```python
from build123d import *

# Parameters (mm, degrees)
SKETCH1_R           = 5.75
BOSS_EXTRUDE1_DEPTH = 7
CUT_EXTRUDE1_DEPTH  = 7
FILLET1_R           = 1
FILLET2_R           = 1
FILLET3_R           = 1
FILLET4_R           = 1
CUT_EXTRUDE2_DEPTH  = 0.5


with BuildPart() as part:
    # Sketch1 → Boss-Extrude1 (new body)
    with BuildSketch(Plane(origin=(0, 0, 0), x_dir=(1, 0, 0), z_dir=(0, 1, 0))):
        with BuildLine():
            Line((-27.5, -15), (27.5, -15))
            ThreePointArc((27.5, -15), (34.571067812, -12.071067812), (37.5, -5))
            Line((37.5, -5), (37.5, 5))
            ThreePointArc((37.5, 5), (34.571067812, 12.071067812), (27.5, 15))
            Line((27.5, 15), (-27.5, 15))
            ThreePointArc((-27.5, 15), (-34.571067812, 12.071067812), (-37.5, 5))
            Line((-37.5, 5), (-37.5, -5))
            ThreePointArc((-37.5, -5), (-34.571067812, -12.071067812), (-27.5, -15))
        make_face()
        with Locations(Location((0, 0, 0), (0, 0, 270))):
            Circle(SKETCH1_R, mode=Mode.SUBTRACT)
    extrude(amount=BOSS_EXTRUDE1_DEPTH)

    # Sketch2 → Cut-Extrude1 (cut)
    with BuildSketch(Plane(origin=(0, 7, 0), x_dir=(1, 0, 0), z_dir=(0, 1, 0))):
        with BuildLine():
            Line((-34.875660829, 0), (-34.571067812, 12.071067812))
            Line((-34.571067812, 12.071067812), (-34.571067812, 15))
            Line((-34.571067812, 15), (-27.5, 15))
            Line((-27.5, 15), (-10.275660829, 15))
            Line((-10.275660829, 15), (-10.275660829, 0))
            ThreePointArc((-10.275660829, 0), (-22.575660829, -12.3), (-34.875660829, 0))
        make_face()
    cut_extrude1 = extrude(amount=-CUT_EXTRUDE1_DEPTH, mode=Mode.SUBTRACT)

    # Fillet1
    fillet1_edges = [part.edges().sort_by_distance(p)[0] for p in [
        (-34.571067812, 3.5, -12.071067812),
    ]]
    fillet(fillet1_edges, radius=FILLET1_R)

    # Fillet2
    fillet2_edges = [part.edges().sort_by_distance(p)[0] for p in [
        (-10.275660829, 3.5, -15),
    ]]
    fillet(fillet2_edges, radius=FILLET2_R)

    # Mirror1: Cut-Extrude1 across plane
    add(cut_extrude1.mirror(Plane.ZY), mode=Mode.SUBTRACT)

    # Fillet3
    fillet3_edges = [part.edges().sort_by_distance(p)[0] for p in [
        (10.275660829, 3.5, -15),
    ]]
    fillet(fillet3_edges, radius=FILLET3_R)

    # Fillet4
    fillet4_edges = [part.edges().sort_by_distance(p)[0] for p in [
        (34.571067812, 3.5, -12.071067812),
    ]]
    fillet(fillet4_edges, radius=FILLET4_R)

    # Sketch3 → Cut-Extrude2 (cut)
    with BuildSketch(Plane.XZ):
        Polygon((0, 10.201614586), (-8.834857391, 5.100807293), (-8.834857391, -5.100807293), (0, -10.201614586), (8.834857391, -5.100807293), (8.834857391, 5.100807293), align=None)
    extrude(amount=-CUT_EXTRUDE2_DEPTH, mode=Mode.SUBTRACT)


solid = part.part
```
Can you work these out from the model? Positions are in its coordinate system, mm. A direction names the side the tool comes from. Coordinates: 2 decimals unless noted, no trailing zeros. Loops run counter-clockwise (first coordinate to the right, second up) from the corner with the lowest first, then second, coordinate; pieces in that order, holes last. Notation, with made-up numbers: (81.5, 28) - (119.5, 28) arc R25 ccw to (119.5, 46) - close; hole circle Ø6 at (77.25, -8). An arc over 180 degrees is marked (long way). Use a Markdown table: item, result.
Item 1: I want a section at C-C on z = -12.25. Please give me the cut outline in (x, y).
Numbers:
| item | result |
|---|---|
| outline | (-10.28, 0) - (10.28, 0) - (10.28, 7) - (-10.28, 7) - close |
Item 2: I want a section at B-B on y = 5.5. Please give me the cut outline in (x, z), and give its area (3 significant figures).
Numbers:
| item | result |
|---|---|
| outline | (-37.5, -5) arc R10 ccw to (-36.56, -9.23) arc R1 ccw to (-34.65, -8.78) - (-34.88, 0) arc R12.3 cw to (-10.28, 0) - (-10.28, -14) arc R1 ccw to (-9.28, -15) - (9.28, -15) arc R1 ccw to (10.28, -14) - (10.28, 0) arc R12.3 cw to (34.88, 0) - (34.65, -8.78) arc R1 ccw to (36.56, -9.23) arc R10 ccw to (37.5, -5) - (37.5, 5) arc R10 ccw to (27.5, 15) - (-27.5, 15) arc R10 ccw to (-37.5, 5) - close; hole circle Ø11.5 at (0, 0) |
| area | 860 mm2 |
Item 3: I want a section at A-A on z = 6.75. Please give me the cut outline in (x, y).
Numbers:
| item | result |
|---|---|
| outline | (-37.35, 0) - (-32.86, 0) - (-32.86, 7) - (-37.35, 7) - close; (-12.29, 0) - (-5.98, 0) - (-5.98, 0.5) - (5.98, 0.5) - (5.98, 0) - (12.29, 0) - (12.29, 7) - (-12.29, 7) - close; (32.86, 0) - (37.35, 0) - (37.35, 7) - (32.86, 7) - close |
Item 4: If I drill on probe 1 along X at (y, z) = (6.25, -2.5); probe 2 along X at (y, z) = (3, -2.75); probe 3 along Z at (x, y) = (0, 3.5), over which ranges is the centre line in solid material (lowest first)? Write a range as from..to.
Numbers:
| item | result |
|---|---|
| probe 1 | x = -37.5..-34.81, -10.28..-5.18, 5.18..10.28, 34.81..37.5 |
| probe 2 | x = -37.5..-34.81, -10.28..-5.05, 5.05..10.28, 34.81..37.5 |
| probe 3 | z = -15..-5.75, 5.75..15 |
Item 5: For faces 1 (the face through (4.479, 0.246, 7.616)), 2 (the face through (-10.276, 4, -7)), 3 (the face through (34.49, 3.45, 12.15)), which set-ups out of +Z, -Z, +X, -X, +Y, -Y let a thin tool reach every point of the face, with its end or its side?
Numbers:
| item | result |
|---|---|
| face 1 | -Y |
| face 2 | -Z, +Y, -Y |
| face 3 | +Z, +X, +Y, -Y |
Item 6: Will this pin go through, and if not, where does the flat tip stop? pin 1 (1 mm diameter, centred on y = 3.5, z = -6, fed in from -X).
Numbers:
| item | result |
|---|---|
| pin 1 | stops at x = -37.49 |
Item 7: I want a section at D-D on x = 7. Please give me the cut outline in (y, z), and give its area (3 significant figures).
Numbers:
| item | result |
|---|---|
| outline | (0, -15) - (7, -15) - (7, 15) - (0, 15) - (0, 6.16) - (0.5, 6.16) - (0.5, -6.16) - (0, -6.16) - close |
| area | 204 mm2 |
Item 8: We'd pull the mould along X, two halves only. Please class faces 4 (the face through (4.85, 3.7, 3.09)), 5 (the face through (0, 3, -15)), 6 (the face through (-34.65, 3.45, 11.99)): released by +X, released by -X, zero draft, split by the parting line, or undercut.
Numbers:
| item | result |
|---|---|
| face 4 | undercut |
| face 5 | zero draft |
| face 6 | released by -X |
